```python
from build123d import *

# Parameters (mm, degrees)
SKETCH1_W                      = 400
SKETCH1_H                      = 400
BOSS_EXTRUDE1_DEPTH            = 3
HOLE1_D                        = 52
HOLE1_DEPTH                    = 10
HOLE2_D                        = 23
HOLE2_DEPTH                    = 100
M4_CLEARANCE_HOLE1_D           = 4.8
M4_CLEARANCE_HOLE1_CSINK_D     = 4.85
M4_CLEARANCE_HOLE1_CSINK_ANGLE = 90
M3_CLEARANCE_HOLE1_D           = 3.6
M3_CLEARANCE_HOLE1_CSINK_D     = 3.65
M3_CLEARANCE_HOLE1_CSINK_ANGLE = 90
SKETCH11_W                     = 667.246369456
SKETCH11_H                     = 555.388303621
CUT_EXTRUDE1_DEPTH             = 1
CUT_EXTRUDE1_DEPTH_BACK        = 4
M3_CLEARANCE_HOLE2_D           = 3.6
M3_CLEARANCE_HOLE2_CSINK_D     = 3.65
M3_CLEARANCE_HOLE2_CSINK_ANGLE = 90


with BuildPart() as part:
    # Sketch1 → Boss-Extrude1 (new body)
    with BuildSketch(Plane(origin=(0, 0, 0), x_dir=(1, 0, 0), z_dir=(0, 1, 0))):
        with Locations((0, -52.110233191)):
            Rectangle(SKETCH1_W, SKETCH1_H)
    extrude(amount=-BOSS_EXTRUDE1_DEPTH)

    # Hole1
    with Locations(Plane(origin=(0, 0, 0), x_dir=(1, 0, 0), z_dir=(0, 1, 0))):
        with Locations((0, 0)):
            Hole(HOLE1_D / 2, depth=HOLE1_DEPTH)

    # Hole2
    with Locations(Plane(origin=(0, 0, 0), x_dir=(1, 0, 0), z_dir=(0, 1, 0))):
        with Locations((0, -107.6)):
            Hole(HOLE2_D / 2, depth=HOLE2_DEPTH)

    # M4 Clearance Hole1 (through all)
    with Locations(Plane(origin=(0, 0, 0), x_dir=(1, 0, 0), z_dir=(0, 1, 0))):
        with Locations((0, -38.6), (33.428580586, 19.3), (-33.428580586, 19.3)):
            CounterSinkHole(M4_CLEARANCE_HOLE1_D / 2, M4_CLEARANCE_HOLE1_CSINK_D / 2, counter_sink_angle=M4_CLEARANCE_HOLE1_CSINK_ANGLE)

    # M3 Clearance Hole1 (through all)
    with Locations(Plane(origin=(0, 0, 0), x_dir=(1, 0, 0), z_dir=(0, 1, 0))):
        with Locations((15.556349186, -92.043650814), (-15.556349186, -92.043650814), (-15.556349186, -123.156349186), (15.556349186, -123.156349186)):
            CounterSinkHole(M3_CLEARANCE_HOLE1_D / 2, M3_CLEARANCE_HOLE1_CSINK_D / 2, counter_sink_angle=M3_CLEARANCE_HOLE1_CSINK_ANGLE)

    # Sketch11 → Cut-Extrude1 (cut, two sides)
    with BuildSketch(Plane(origin=(0, 0, 0), x_dir=(1, 0, 0), z_dir=(0, 1, 0))) as cut_extrude1_sk:
        with Locations((-28.870236031, -19.694924611)):
            Rectangle(SKETCH11_W, SKETCH11_H)
        with BuildLine():
            Line((-46.718297015, -86.518), (-76.718297015, -86.518))
            ThreePointArc((-76.718297015, -86.518), (-91.287101954, -80.220186783), (-96.680745664, -65.292992264))
            Line((-96.680745664, -65.292992264), (-92.326325, 5.665660778))
            ThreePointArc((-92.326325, 5.665660778), (0, 92.5), (92.326325, 5.665660778))
            Line((92.326325, 5.665660778), (96.680745664, -65.292992264))
            ThreePointArc((96.680745664, -65.292992264), (96.708906973, -65.905208425), (96.718297015, -66.518))
            ThreePointArc((96.718297015, -66.518), (90.860432639, -80.660135624), (76.718297015, -86.518))
            Line((76.718297015, -86.518), (46.718297015, -86.518))
            ThreePointArc((46.718297015, -86.518), (37.114124402, -91.017383247), (34.424008327, -101.276421053))
            ThreePointArc((34.424008327, -101.276421053), (34.855704637, -104.425121376), (35, -107.6))
            ThreePointArc((35, -107.6), (-3.174878624, -142.455704637), (-34.424008327, -101.276421053))
            ThreePointArc((-34.424008327, -101.276421053), (-37.114124402, -91.017383247), (-46.718297015, -86.518))
        make_face(mode=Mode.SUBTRACT)
    extrude(amount=CUT_EXTRUDE1_DEPTH, mode=Mode.SUBTRACT)
    extrude(cut_extrude1_sk.sketch, amount=-CUT_EXTRUDE1_DEPTH_BACK, mode=Mode.SUBTRACT)

    # M3 Clearance Hole2 (through all)
    with Locations(Plane(origin=(0, 0, 0), x_dir=(1, 0, 0), z_dir=(0, 1, 0))):
        with Locations((-64.951905284, 37.5), (0, -75), (64.951905284, 37.5)):
            CounterSinkHole(M3_CLEARANCE_HOLE2_D / 2, M3_CLEARANCE_HOLE2_CSINK_D / 2, counter_sink_angle=M3_CLEARANCE_HOLE2_CSINK_ANGLE)


solid = part.part
```
Geometry: final body of the model. Coordinates: model frame, mm. Coordinates: 2 decimals unless noted, no trailing zeros. Order: outer loops, then holes, each group sorted by start corner. A loop starts at its lowest first (then second) coordinate and runs counter-clockwise, first axis right, second up.
Item 1: Draft query along Z for faces 1 (the face through (-1.95, -1.48, -92.48)), 2 (the face through (0.31, -1.53, 36.22)), 3 (the face through (-23, 0, 23)). Return one class per face: released by +Z, released by -Z, zero draft, split by the parting line, or undercut.
Answer:
face 1: released by -Z
face 2: undercut
face 3: zero draft
Item 2: Contact query for flat-ended pins moving along their axis: P1, Ø14, axis at x = 0, z = 107.6, coming from the +Y side; P2, Ø4, axis at x = -64.95, z = -37.5, coming from the -Y side; P3, Ø1.5, axis at x = 57, y = -1, coming from the +Z side. Output: stop coordinate, or through.
Answer:
P1: passes through
P2: stops at y = -3
P3: stops at z = 86.52
Item 3: Section query C-C (x = 55.5). Output: boundary loops of the cut face in (y, z), then the cut area to 3 significant figures.
Answer:
outline: (-3, -74) - (0, -74) - (0, 86.52) - (-3, 86.52) - close
area: 482 mm2
Item 4: Material intervals for line 1 along Z through (x, y) = (0, -1.9); line 2 along X through (y, z) = (-0.7, -36.5); line 3 along X through (y, z) = (-2.7, 91), sorted ascending.
Answer:
line 1: z = -92.5 to -26, 26 to 36.2, 41 to 73.2, 76.8 to 96.1, 119.1 to 142.6
line 2: x = -84.99 to -66.45, -63.46 to 63.46, 66.45 to 84.99
line 3: x = -37.13 to -17.02, -14.09 to 14.09, 17.02 to 37.13
Item 5: Section query A-A (z = 0). Output: boundary loops of the cut face in (x, y), then the cut area to 3 significant figures.
Answer:
outline: (-92.67, -3) - (-26, -3) - (-26, 0) - (-92.67, 0) - close; (26, -3) - (92.67, -3) - (92.67, 0) - (26, 0) - close
area: 400 mm2
Item 6: Section query D-D (z = -78). Output: boundary loops of the cut face in (x, y), then the cut area to 3 significant figures.
Answer:
outline: (-49.72, -3) - (49.72, -3) - (49.72, 0) - (-49.72, 0) - close
area: 298 mm2
Item 7: Section query B-B (y = -0.7). State how many separate pieces and enclosed holes the cut face has, then the cut area to 3 significant figures.
Answer:
separate pieces: 1
enclosed holes: 12
area: 30,500 mm2
